Design review of the part built by this model. Coordinates are the model's own, in mm. A direction names the side the tool comes from. Give positions to 0.01 mm unless a question says otherwise; leave off trailing zeros. Loops run counter-clockwise (first coordinate to the right, second up) from the corner with the lowest first, then second, coordinate; pieces in that order, holes last. Notation, with made-up numbers: M 32.5,16 L 47.5,16 A8 ccw 47.5,24 Z; hole C 0,-33 d4. An arc over 180 degrees is marked long. Use CSV: the item, a comma, the result in double quotes.
from build123d import *

# Parameters (mm, degrees)
SKETCH_1_R      = 1.6
SKETCH_1_R_2    = 12
EXTRUDE_1_DEPTH = 5
SKETCH_4_W      = 42
SKETCH_4_H      = 50
SKETCH_4_R      = 1.6
EXTRUDE_4_DEPTH = 5
FILLET_1_R      = 2


with BuildPart() as part:
    # 草图1 → 凸台-拉伸1 (new body)
    with BuildSketch(Plane(origin=(0, 0, 0), x_dir=(1, 0, 0), z_dir=(0, 1, 0))):
        Polygon((-21, -21), (-21, 21), (21, 21), (21, -21), (21, -23), (-21, -23), align=None)
        with Locations(Location((-15.5, 15.5, 0), (0, 0, 270))):
            Circle(SKETCH_1_R, mode=Mode.SUBTRACT)
        with Locations(Location((15.5, 15.5, 0), (0, 0, 270))):
            Circle(SKETCH_1_R, mode=Mode.SUBTRACT)
        with Locations(Location((-15.5, -15.5, 0), (0, 0, 270))):
            Circle(SKETCH_1_R, mode=Mode.SUBTRACT)
        with Locations(Location((15.5, -15.5, 0), (0, 0, 270))):
            Circle(SKETCH_1_R, mode=Mode.SUBTRACT)
        with Locations(Location((0, 0, 0), (0, 0, 270))):
            Circle(SKETCH_1_R_2, mode=Mode.SUBTRACT)
    extrude(amount=EXTRUDE_1_DEPTH)

    # 草图4 → 凸台-拉伸4 (add)
    with BuildSketch(Plane.XY.offset(23)):
        with Locations((0, 25)):
            Rectangle(SKETCH_4_W, SKETCH_4_H)
        with Locations((-15.5, 44.5)):
            Circle(SKETCH_4_R, mode=Mode.SUBTRACT)
        with Locations((15.5, 44.5)):
            Circle(SKETCH_4_R, mode=Mode.SUBTRACT)
        with Locations((-15.5, 13.5)):
            Circle(SKETCH_4_R, mode=Mode.SUBTRACT)
        with Locations((15.5, 13.5)):
            Circle(SKETCH_4_R, mode=Mode.SUBTRACT)
    extrude(amount=EXTRUDE_4_DEPTH)

    # 圆角1
    fillet_1_edges = [part.edges().sort_by_distance(p)[0] for p in [
        (0, 5, 23),
    ]]
    fillet(fillet_1_edges, radius=FILLET_1_R)


solid = part.part
(1) Clearance check with flat-ended pins moving along their axes: P1, Ø5, axis at x = 12, z = 2, coming from the -Y side; P2, Ø5, axis at x = -15.5, y = 13.5, coming from the -Z side; P3, Ø21, axis at x = 3, z = 7, coming from the +Y side. State where each tip first meets the part, or that it passes through.
A:
P1,"y = 0"
P2,"z = 23"
P3,"y = 5"
(2) We need section B-B on z = 0. State the section outline as (x, y) points.
A:
outline,"M -21,0 L -12,0 L -12,5 L -21,5 Z; M 12,0 L 21,0 L 21,5 L 12,5 Z"
(3) Wall thickness on line 1 along X through (y, z) = (3.95, 15.5); line 2 along Y through (x, z) = (-15.5, 25.1); line 3 along X through (y, z) = (3, 15): over which ranges is each line inside the solid? List them lowest first. Write a range as [from, to].
A:
line 1,"[-21, -17.1], [-13.9, 13.9], [17.1, 21]"
line 2,"[0, 11.9], [15.1, 42.9], [46.1, 50]"
line 3,"[-21, -17.02], [-13.98, 13.98], [17.02, 21]"
(4) The part is to be moulded in two halves that separate along Z. For faces 1 (the cylindrical face through (3.604, 2.465, 11.446)), 2 (the cylindrical face through (16.58, 2.46, 14.32)), 3 (the cylindrical face through (14.23, 43.53, 25.46)), 4 (the flat face through (0, 2, -21)), say which applies: released by +Z, released by -Z, zero draft, split by the parting line, or undercut.
A:
face 1,"undercut"
face 2,"undercut"
face 3,"zero draft"
face 4,"released by -Z"
(5) Machinability: for faces 5 (the flat face through (10, 5, -10)), 6 (the cylindrical face through (-16.68, 14.58, 25.46)), which of the approach directions +Z, -Z, +X, -X, +Y, -Y give a long, thin tool a straight path to every point of the face, cutting with its end or side? Answer none if there is none.
A:
face 5,"-Z, +X, -X, +Y"
face 6,"+Z, -Z"
(6) We need section D-D on x = 0. State the section outline as (y, z) points.
A:
outline,"M 0,-21 L 5,-21 L 5,-12 L 0,-12 Z; M 0,12 L 5,12 L 5,21 A2 cw 7,23 L 50,23 L 50,28 L 0,28 Z"
(7) We need section A-A on x = -15.5. State the section outline as (y, z) points.
A:
outline,"M 0,-21 L 5,-21 L 5,-17.1 L 0,-17.1 Z; M 0,-13.9 L 5,-13.9 L 5,13.9 L 0,13.9 Z; M 0,17.1 L 5,17.1 L 5,21 A2 cw 7,23 L 11.9,23 L 11.9,28 L 0,28 Z; M 15.1,23 L 42.9,23 L 42.9,28 L 15.1,28 Z; M 46.1,23 L 50,23 L 50,28 L 46.1,28 Z"
(8) We need section C-C on y = 13.5. State the section outline as (x, z) points.
A:
outline,"M -21,23 L -17.1,23 L -17.1,28 L -21,28 Z; M -13.9,23 L 13.9,23 L 13.9,28 L -13.9,28 Z; M 17.1,23 L 21,23 L 21,28 L 17.1,28 Z"
